from build123d import *

# Parameters (mm, degrees)
BOSS_EXTRUDE1_DEPTH = 81
BOSS_EXTRUDE2_DEPTH = 2


with BuildPart() as part:
    # Sketch1 → Boss-Extrude1 (new body)
    with BuildSketch(Plane(origin=(0, 0, 0), x_dir=(1, 0, 0), z_dir=(0, 1, 0))):
        Polygon((23.002372201, -47.057873482), (-38.997627799, -47.057873482), (-18.264673723, 8.930513794), (-38.588834845, 116.906230278), (-10.371463192, 116.906230278), (23.002372201, 14.192126518), align=None)
        Polygon((-36.1242874, -45.057873482), (21.002372201, -45.057873482), (21.002372201, 13.875357637), (-11.824548248, 114.906230278), (-36.177255073, 114.906230278), (-16.196659594, 8.755767302), align=None, mode=Mode.SUBTRACT)
    extrude(amount=BOSS_EXTRUDE1_DEPTH)

    # Sketch2 → Boss-Extrude2 (add)
    with BuildSketch(Plane(origin=(0, 81, 0), x_dir=(1, 0, 0), z_dir=(0, 1, 0))):
        Polygon((-38.997627799, -47.057873482), (23.002372201, -47.057873482), (23.002372201, 14.192126518), (-10.371463192, 116.906230278), (-38.588834845, 116.906230278), (-18.264673723, 8.930513794), align=None)
    extrude(amount=BOSS_EXTRUDE2_DEPTH)


solid = part.part
Can you work these out from the model? Positions are in its coordinate system, mm. A direction names the side the tool comes from. Give positions to 0.01 mm unless a question says otherwise; leave off trailing zeros. Order: outer loops, then holes, each group sorted by start corner. A loop starts at its lowest first (then second) coordinate and runs counter-clockwise, first axis right, second up. Notation, with made-up numbers: M 86.25,-28 L 132.25,-28 A19 cw 132.25,8 Z; hole C 45.5,27 d10. An arc over 180 degrees is marked long. One line per item, written item: value.
Item 1: If we section it at B-B on y = 53: Write out the boundary of the cut face in (x, z).
Verdict:
outline: M -39,47.06 L -18.26,-8.93 L -38.59,-116.91 L -10.37,-116.91 L 23,-14.19 L 23,47.06 Z; hole M -36.18,-114.91 L -11.82,-114.91 L 21,-13.88 L 21,45.06 L -36.12,45.06 L -16.2,-8.76 Z
Item 2: Please list where these lines run through material, in increasing order: line 1 (Y direction, x = -23.5, z = -87.5); line 2 (X direction, y = 52, z = -25.5); line 3 (X direction, y = 40, z = 40.5).
Verdict:
line 1: 81 to 83
line 2: -21.38 to -19.35, 17.23 to 19.33
line 3: -36.57 to -34.44, 21 to 23
Item 3: For pin 1 (1 mm diameter, centred on y = 25.5, z = -79.5, fed in from +X) (3 decimals); pin 2 (1.5 mm diameter, centred on y = 18.5, z = 21.5, fed in from -X); pin 3 (1 mm diameter, centred on y = 49.5, z = -55.5, fed in from -X), each with a flat end and sliding along its axis, tell me the tip position at first contact or that it passes through.
Verdict:
pin 1: x = 1.945
pin 2: x = -29.81
pin 3: x = -27.12
Item 4: If we section it at A-A on x = -29: Write out the boundary of the cut face in (y, z), and give its area (3 significant figures).
Verdict:
outline: M 0,-116.91 L 83,-116.91 L 83,-65.96 L 0,-65.96 L 0,-76.78 L 81,-76.78 L 81,-114.91 L 0,-114.91 Z; M 0,20.06 L 83,20.06 L 83,47.06 L 0,47.06 L 0,45.06 L 81,45.06 L 81,25.82 L 0,25.82 Z
area: 1,820 mm2
Item 5: If we section it at C-C on z = -88.5: Write out the boundary of the cut face in (x, y).
Verdict:
outline: M -33.24,0 L -31.21,0 L -31.21,81 L -3.24,81 L -3.24,0 L -1.14,0 L -1.14,83 L -33.24,83 Z
Item 6: If we mould it in two halves opening along Z, with no side actions, what happens to faces 4 (the face through (6.55, 40.92, -64.83)), 5 (the face through (-22, 0, -35)), 6 (the face through (21.002, 40, 16)), 7 (the face through (-8, 41, 47.058))? For each: pulls with the +Z half, pulls with the -Z half, needs draft (parallel to the pull), parting line crosses it, or undercut.
Verdict:
face 4: pulls with the -Z half
face 5: needs draft
face 6: undercut
face 7: pulls with the +Z half
Item 7: For faces 1 (the face through (-8, 83, -36)), 2 (the face through (-28.57, 40.92, -63.67)), 3 (the face through (-26.327, 39.933, -62.574)), which set-ups out of +Z, -Z, +X, -X, +Y, -Y let a thin tool reach every point of the face, with its end or its side?
Verdict:
face 1: +Z, -Z, +X, -X, +Y
face 2: -X, +Y, -Y
face 3: -Y
Item 8: If we section it at D-D on x = -7: Write out the boundary of the cut face in (y, z).
Verdict:
outline: M 0,-106.53 L 83,-106.53 L 83,47.06 L 0,47.06 L 0,45.06 L 81,45.06 L 81,-100.06 L 0,-100.06 Z
